Autodesk Inventor part; units mm, degrees
ref_plane "YZ Plane" through (0, 0, 0) normal (1, 0, 0) x (0, 1, 0)
ref_plane "XZ Plane" through (0, 0, 0) normal (0, 1, 0) x (-1, 0, 0)
ref_plane "XY Plane" through (0, 0, 0) normal (0, 0, 1) x (1, 0, 0)
sketch "Sketch1" plane through (0, 0, 0) normal (0, 0, 1) x (1, 0, 0)
  line L0 (-490, 64) -> (490, 64)
  line L1 (490, 64) -> (490, 0)
  line L2 (490, 0) -> (-490, 0)
  line L3 (-490, 0) -> (-490, 64)
  point P0 (0, 0)
  point P1 (0, 0)
  dimension "d0" = 980
  dimension "d1" = 64
extrude "Plate1" add sketch "Sketch1" along normal blind 2
sketch "Sketch2" plane through (490, 2, 0) normal (0, -1, 0) x (1, 0, 0)
  line L0 (-980, 0) -> (0, 0)
  line L1 (0, 0) -> (0, 20)
  line L2 (0, 20) -> (-980, 20)
  line L3 (-980, 20) -> (-980, 0)
edge flange "Flange1" height 20 angle 90 thickness 2 bend radius 2.75 thickness toward (0, -1, 0) relief round relief width 2 relief depth 1 edges at (0, 0, 2) wall of the first edge with corners at (-490, 2, 0) (490, 2, 0) (490, 2, 20) (-490, 2, 20)
bend "Bend1"
corner "Corner1"
sketch "Sketch5" plane through (0, 0, 0) normal (0, 0, -1) x (-1, 0, 0)
  line L0 (490, 64) -> (-490, 64)
  line L1 (490, 0) -> (-490, 0)
  circle A0 centre (0, 64) radius 35
  line L2 (243.95, 64) -> (246.05, 64)
  line L3 (246.05, 64) -> (246.05, 29)
  line L4 (246.05, 29) -> (243.95, 29)
  line L5 (243.95, 29) -> (243.95, 64)
  line L6 (-243.95, 64) -> (-246.05, 64)
  line L7 (-246.05, 64) -> (-246.05, 29)
  line L8 (-246.05, 29) -> (-243.95, 29)
  line L9 (-243.95, 29) -> (-243.95, 64)
  line L10 (0, 64) -> (0, 0) construction
  line L11 (-490, 0) -> (-490, 64)
  line L12 (490, 0) -> (490, 64)
  circle A1 centre (-490, 64) radius 35
  circle A2 centre (490, 64) radius 35
  point P0 (0, 0)
  point P1 (245, 29)
  point P2 (-245, 29)
  point P3 (246.05, 64)
  point P4 (-35, 64)
  point P5 (35, 64)
  point P6 (-246.05, 64)
  point P7 (455, 64)
  point P8 (490, 29)
  point P9 (-490, 29)
  point P10 (-455, 64)
  dimension "d45" = 70
  dimension "d48" = 2.1
  dimension "d49" = 490
  dimension "d51" = 29
  dimension "d52" = 35
extrude "Extrusion1" cut sketch "Sketch5" against normal through all contours L3 L4 L5 L0 | L0 L12 A2 | L9 L8 L7 L0 | L11 L0 A1 picked at (487.4039, 40.9592) picked at (-466.9592, 61.4039)
sketch "Sketch9" plane through (0, 0, 2) normal (0, 0, 1) x (1, 0, 0)
  line L0 (467.0539, 27.7998) -> (467.0539, 15.7998) construction
  line L1 (467.0539, 15.7998) -> (267.0539, 15.7998) construction
  line L2 (267.0539, 15.7998) -> (267.0539, 27.7998) construction
  line L3 (267.0539, 27.7998) -> (467.0539, 27.7998) construction
  line L4 (-490, 64) -> (490, 64)
  point P0 (0, 0)
  point P1 (1.05, 68)
  point P2 (490, 64)
  point P3 (-490, 64)
  dimension "d40" = 200
  dimension "d41" = 12
mark "Mark2"
equation "\"d2\" = Thickness"
equation "\"d3\" = BendReliefWidth"
equation "\"d4\" = BendReliefDepth"
equation "\"d5\" = MinimumRemnant"
equation "\"d6\" = TransitionRadius"
equation "\"d9\" = BendRadius"
equation "\"d10\" = CornerReliefSize"
equation "\"d11\" = GapSize"
equation "\"d12\" = JacobiRadiusSize"
equation "\"BendReliefWidth\" = Thickness"
equation "\"BendReliefDepth\" = 0.5 * Thickness"
equation "\"CornerReliefSize\" = 4 * Thickness"
equation "\"MinimumRemnant\" = 2 * Thickness"
equation "\"TransitionRadius\" = BendRadius"
equation "\"JacobiRadiusSize\" = BendRadius"
equation "\"GapSize\" = Thickness"
properties part number "MSC 309 stringer BOARD  ####" material "Stainless Steel"
Geometry check sheet. Reference: the model listing, model coordinates, mm. A direction names the side the tool comes from. Give positions to 0.01 mm unless a question says otherwise; leave off trailing zeros. Order: outer loops, then holes, each group sorted by start corner. A loop starts at its lowest first (then second) coordinate and runs counter-clockwise, first axis right, second up.
1. Gauge pin test, flat ends, axial feed: pin 1 Ø1 at (y, z) = (52, 1) entering from -X; pin 2 Ø1 at (x, z) = (-245.5, 0.5) entering from +Y; pin 3 Ø12 at (x, z) = (-263.5, 9.5) entering from -Y; pin 4 Ø1.6 at (y, z) = (52, 0.5) entering from +X. Record the tip position at first contact, or that the pin passes through.
2. Access from +Z, -Z, +X, -X, +Y, -Y to the whole of each face (thin tool, end or side, straight path). Record for faces 1 (the face through (-490, 9, 1)), 2 (the face through (7, 2, 12)).
3. Section check B-B, the plane y = 16. Enter the section's corners in (x, z), and give its area (3 significant figures).
4. Thickness scan on L1, parallel to Y at x = -340, z = 12.75; L2, parallel to X at y = 54, z = 1.5. Record the ranges inside material, lowest first.
5. Section check A-A, the plane x = -327. Enter the section's corners in (y, z), and give its area (3 significant figures).
Values follow:
1. pin 1: stops at x = -457.31
1. pin 2: stops at y = 29
1. pin 3: stops at y = 0
1. pin 4: stops at x = 457.42
2. face 1: +Z, -Z, -X, +Y, -Y
2. face 2: +Z, +X, -X, +Y
3. outline: (-490, 0) - (490, 0) - (490, 2) - (-490, 2) - close
3. area: 1,960 mm2
4. L1: y = 0 to 2
4. L2: x = -456.46 to -246.05, -243.95 to 243.95, 246.05 to 456.46
5. outline: (0, 4.75) arc R4.75 ccw to (4.75, 0) - (64, 0) - (64, 2) - (4.75, 2) arc R2.75 cw to (2, 4.75) - (2, 20) - (0, 20) - close
5. area: 161 mm2
